```python
from build123d import *

# Parameters (mm, degrees)
SKETCH1_R                     = 2.75
BOSS_EXTRUDE1_DEPTH           = 10
SKETCH3_R                     = 2
CUT_EXTRUDE1_DEPTH            = 32.5
ESBO_O1_R                     = 2
RESSALTO_EXTRUS_O2_DEPTH      = 13
RESSALTO_EXTRUS_O2_DEPTH_BACK = 3
CORTE_EXTRUS_O1_DEPTH         = 5
FILETE1_R                     = 0.2
FILETE2_R                     = 0.25
CHAMFER_1_SIZE                = 0.3
FILLET_1_R                    = 0.3


with BuildPart() as part:
    # Sketch1 → Boss-Extrude1 (new body)
    with BuildSketch(Plane(origin=(0, 0, 0), x_dir=(1, 0, 0), z_dir=(0, 1, 0))):
        with BuildLine():
            Line((21.5, 0.100660355), (21.5, -0.100660355))
            ThreePointArc((21.5, -0.100660355), (20.891804651, -2.072326113), (19.278590937, -3.35875876))
            Line((19.278590937, -3.35875876), (10, -7))
            Line((10, -7), (10, -14))
            Line((10, -14), (0.5, -14))
            Line((0.5, -14), (0.5, -3.968626967))
            ThreePointArc((0.5, -3.968626967), (0, 4), (-0.5, -3.968626967))
            Line((-0.5, -3.968626967), (-0.5, -14))
            Line((-0.5, -14), (-10, -14))
            Line((-10, -14), (-10, -7))
            Line((-10, -7), (-19.278590937, -3.35875876))
            ThreePointArc((-19.278590937, -3.35875876), (-20.891804651, -2.072326113), (-21.5, -0.100660355))
            Line((-21.5, -0.100660355), (-21.5, 0.100660355))
            ThreePointArc((-21.5, 0.100660355), (-20.881804225, 2.086914218), (-19.245597481, 3.371514512))
            Line((-19.245597481, 3.371514512), (-3.558849946, 9.345297591))
            ThreePointArc((-3.558849946, 9.345297591), (0, 10), (3.558849946, 9.345297591))
            Line((3.558849946, 9.345297591), (19.245597481, 3.371514512))
            ThreePointArc((19.245597481, 3.371514512), (20.881804225, 2.086914218), (21.5, 0.100660355))
        make_face()
        with Locations(Location((-16, 0, 0), (0, 0, 270))):  # turned: the seam where the file's is
            Circle(SKETCH1_R, mode=Mode.SUBTRACT)
        with Locations(Location((16, 0, 0), (0, 0, 270))):  # turned: the seam where the file's is
            Circle(SKETCH1_R, mode=Mode.SUBTRACT)
    extrude(amount=BOSS_EXTRUDE1_DEPTH)

    # Sketch3 → Cut-Extrude1 (cut, through all)
    with BuildSketch(Plane(origin=(10, 0, 0), x_dir=(0, 0, -1), z_dir=(1, 0, 0))):
        with Locations((-10.5, 5)):
            Circle(SKETCH3_R)
    extrude(amount=-CUT_EXTRUDE1_DEPTH, mode=Mode.SUBTRACT)

    # Esboço1 → Ressalto-extrusão2 (add, two sides)
    with BuildSketch(Plane.ZY.offset(-10)) as ressalto_extrus_o2_sk:
        with Locations(Location((10.5, 5, 0), (0, 0, 180))):  # turned: the seam where the file's is
            Circle(ESBO_O1_R)
    extrude(amount=RESSALTO_EXTRUS_O2_DEPTH)
    extrude(ressalto_extrus_o2_sk.sketch, amount=-RESSALTO_EXTRUS_O2_DEPTH_BACK)

    # Esboço2 → Corte-extrusão1 (cut)
    with BuildSketch(Plane.ZY.offset(-13)):
        Polygon((10.90776936, 4.293722751), (11.315538719, 5), (10.90776936, 5.706277249), (10.09223064, 5.706277249), (9.684461281, 5), (10.09223064, 4.293722751), align=None)
    extrude(amount=CORTE_EXTRUS_O1_DEPTH, mode=Mode.SUBTRACT)

    # Filete1
    filete1_edges = [part.edges().sort_by_distance(p)[0] for p in [
        (13, 5, 12.5),
        (13, 4.646861376, 11.11165404),
        (13, 4.293722751, 10.5),
        (13, 4.646861376, 9.88834596),
        (13, 5.353138624, 9.88834596),
        (13, 5.706277249, 10.5),
        (13, 5.353138624, 11.11165404),
    ]]
    fillet(filete1_edges, radius=FILETE1_R)

    # Filete2
    filete2_edges = [part.edges().sort_by_distance(p)[0] for p in [
        (-3, 5, 12.5),
    ]]
    fillet(filete2_edges, radius=FILETE2_R)

    # Фаска1
    chamfer_1_edges = [part.edges().sort_by_distance(p)[0] for p in [
        (0, 0, -4),
        (-16, 0, -2.75),
        (0, 10, -4),
        (-16, 10, -2.75),
        (16, 0, -2.75),
        (16, 10, -2.75),
    ]]
    chamfer(chamfer_1_edges, length=CHAMFER_1_SIZE)

    # Скругление1
    fillet_1_edges = [part.edges().sort_by_distance(p)[0] for p in [
        (10, 5, 14),
        (-10, 5, 14),
    ]]
    fillet(fillet_1_edges, radius=FILLET_1_R)


solid = part.part
```
Here's how the part is built. I have some questions about the finished solid (model axes, mm). A direction names the side the tool comes from. Round coordinates to 2 decimals unless told otherwise and drop trailing zeros. Write each loop counter-clockwise with the first axis right and the second up, starting at its lowest first coordinate (ties: lowest second). Pieces come first, ordered by that corner, then holes. Notation, with made-up numbers: M 67,-27.5 L 102,-27.5 A17 cw 102,1.5 Z; hole C 48.25,-3 d8. An arc over 180 degrees is marked long. Answer as CSV lines item,"result". Start each with the question number.
1. Thinking about a two-plate mould opening in Y: for faces 1 (the cylindrical face through (-6.578, 5.088, 12.498)), 2 (the flat face through (10.4, 5.706, 10.5)), 3 (the cylindrical face through (18.727, 4.934, -0.358)), 4 (the flat face through (-4, 10, 2)), which applies, released by +Y, released by -Y, zero draft, split by the parting line, or undercut?
2. I need wall thicknesses on probe 1 along X at (y, z) = (3, 0); probe 2 along X at (y, z) = (6, 8); probe 3 along X at (y, z) = (5.5, 9.5). Which ranges of each line are inside material? Lowest first, please.
3. Suppose I cut it at B-B on x = 0. Write out the boundary of the cut face in (y, z), then the cut area to 3 significant figures.
4. On a 3-axis mill with a long thin cutter (end or side, diameter ignored), from which of +Z, -Z, +X, -X, +Y, -Y can I reach the whole of each face in a straight line? I mean faces 5 (the cylindrical face through (-20.875, 4.93, 2.096)), 6 (the flat face through (-0.5, 5, 8)), 7 (the flat face through (8, 5, 10)), 8 (the flat face through (-3, 5, 11)), 9 (the cylindrical face through (0, 5, -10)). Say none if no direction works.
5. Suppose I cut it at A-A on y = 8.5. Write out the boundary of the cut face in (x, z).
6. I'm going to push flat-ended pins straight in: pin 1 Ø1.5 at (x, y) = (-8.5, 2.5) entering from -Z; pin 2 Ø5 at (x, y) = (-15, 7) entering from -Z; pin 3 Ø3.5 at (y, z) = (4.5, 9) entering from -X; pin 4 Ø6.5 at (x, z) = (16, 0) entering from -Y. Where does each tip first touch, or does it pass through?
7. Suppose I cut it at C-C on z = 5.25. Write out the boundary of the cut face in (x, y).
Check result:
1,face 1,"undercut"
1,face 2,"undercut"
1,face 3,"zero draft"
1,face 4,"released by +Y"
2,probe 1,"x = -21.5 to -18.75, -13.25 to -4, 4 to 13.25, 18.75 to 21.5"
2,probe 2,"x = -10 to -0.5, 0.5 to 10"
2,probe 3,"x = -3 to 13"
3,outline,"M 0,-10 L 10,-10 L 10,-4.3 L 9.7,-4 L 0.3,-4 L 0,-4.3 Z; C 5,10.5 d4"
3,area,"72.5 mm2"
4,face 5,"+Z, -X, +Y, -Y"
4,face 6,"none"
4,face 7,"+X"
4,face 8,"-X"
4,face 9,"-Z, +Y, -Y"
5,outline,"M -21.5,-0.1 A3.5 ccw -19.25,-3.37 L -3.56,-9.35 A10 ccw 3.56,-9.35 L 19.25,-3.37 A3.5 ccw 21.5,-0.1 L 21.5,0.1 A3.5 ccw 19.28,3.36 L 10,7 L 10,13.7 A0.3 ccw 9.7,14 L 0.5,14 L 0.5,3.97 A4 cw long -0.5,3.97 L -0.5,14 L -9.7,14 A0.3 ccw -10,13.7 L -10,7 L -19.28,3.36 A3.5 ccw -21.5,0.1 Z; hole C -16,0 d5.5; hole C 16,0 d5.5"
6,pin 1,"stops at z = -7.75"
6,pin 2,"stops at z = -5.94"
6,pin 3,"stops at x = -10"
6,pin 4,"stops at y = 0"
7,outline,"M -14.46,0 L -0.5,0 L -0.5,10 L -14.46,10 Z; M 0.5,0 L 14.46,0 L 14.46,10 L 0.5,10 Z"
